Input: dimensioned drawing with shaded views. Units: mm. Origin: part minimum x, y, z. A direction names the side the tool comes from. Round coordinates to 2 decimals unless told otherwise and drop trailing zeros. Loops run counter-clockwise (first coordinate to the right, second up) from the corner with the lowest first, then second, coordinate; pieces in that order, holes last. Notation, with made-up numbers: M 9,33.5 L 38,33.5 A28 cw 38,65.5 Z; hole C -37.5,88.5 d7. An arc over 180 degrees is marked long. Write each question's results on one line, items separated by ' | '. Start each with the question number.
1. Section D-D on x = 5. Output: boundary loops of the cut face in (y, z) (1 decimal).
2. Set-up query: the marked faces 1 and 2. Return all of +Z, -Z, +X, -X, +Y, -Y with unobstructed straight access to the full face (end or side cutting, diameter ignored); none if empty.
3. Contact query for a flat-ended pin moving along its axis: pin 1 Ø4.5 at (y, z) = (25.4, 38.1) entering from +X (1 decimal). Output: stop coordinate, or through.
4. Ray query, line 1 (Y direction, x = 24.5, z = 12.7); line 2 (Y direction, x = 5.5, z = 31) (1 decimal); line 3 (X direction, y = 37, z = 49) (1 decimal). Return the intervals inside material, ascending.
5. Draft query along X for the marked faces 3, 4, 5 and 6. Return one class per face: released by +X, released by -X, zero draft, split by the parting line, or undercut.
6. Section C-C on z = 38.1. Output: boundary loops of the cut face in (x, y) (1 decimal), and give its area (3 significant figures).
7. Section A-A on z = 12.7. Output: boundary loops of the cut face in (x, y) (1 decimal), and give its area (3 significant figures).
8. Section B-B on y = 25.4. Output: boundary loops of the cut face in (x, z) (1 decimal).
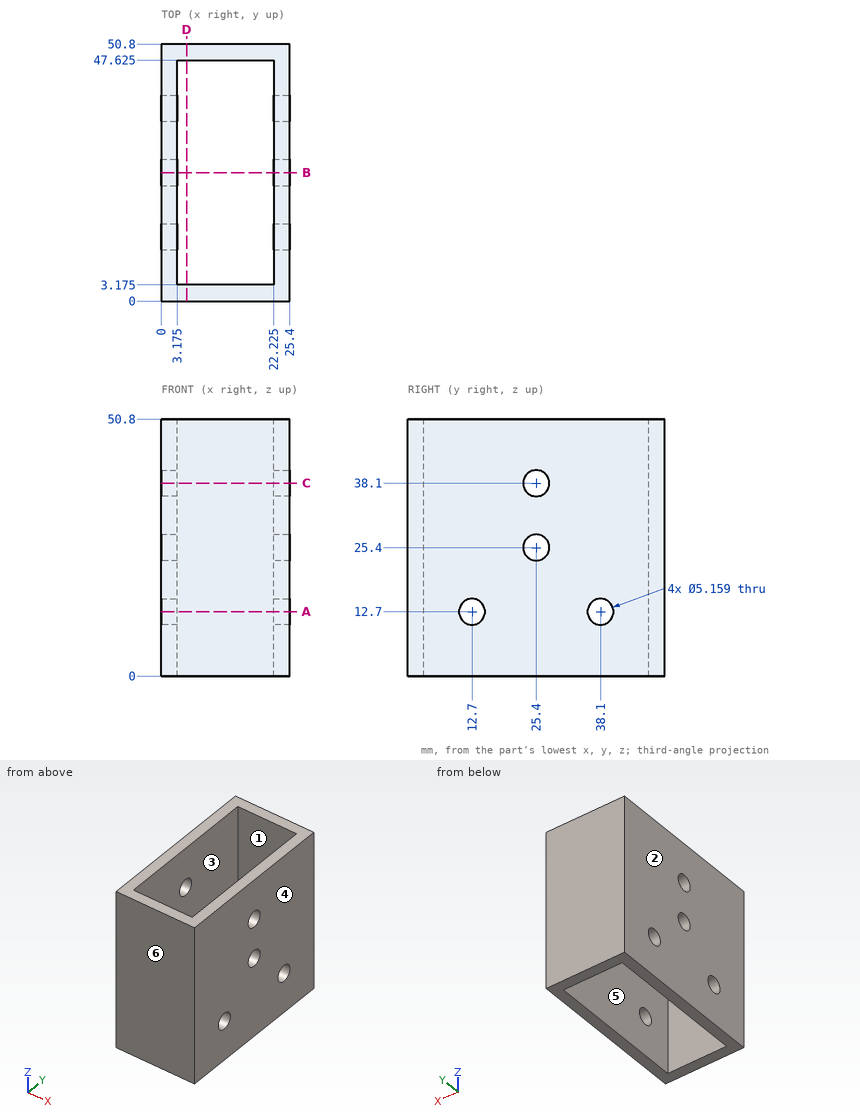
Taken from the geometry:
1) outline: M 0,0 L 3.2,0 L 3.2,50.8 L 0,50.8 Z; M 47.6,0 L 50.8,0 L 50.8,50.8 L 47.6,50.8 Z
2) face 1: +Z, -Z | face 2: +Z, -Z, -X, +Y, -Y
3) pin 1: through
4) line 1: 0 to 10.12, 15.28 to 35.52, 40.68 to 50.8 | line 2: 0 to 3.2, 47.6 to 50.8 | line 3: 0 to 3.2, 22.2 to 25.4
5) face 3: undercut | face 4: released by +X | face 5: undercut | face 6: zero draft
6) outline: M 0,0 L 25.4,0 L 25.4,22.8 L 22.2,22.8 L 22.2,3.2 L 3.2,3.2 L 3.2,22.8 L 0,22.8 Z; M 0,28 L 3.2,28 L 3.2,47.6 L 22.2,47.6 L 22.2,28 L 25.4,28 L 25.4,50.8 L 0,50.8 Z | area: 411 mm^2
7) outline: M 0,0 L 25.4,0 L 25.4,10.1 L 22.2,10.1 L 22.2,3.2 L 3.2,3.2 L 3.2,10.1 L 0,10.1 Z; M 0,15.3 L 3.2,15.3 L 3.2,35.5 L 0,35.5 Z; M 0,40.7 L 3.2,40.7 L 3.2,47.6 L 22.2,47.6 L 22.2,40.7 L 25.4,40.7 L 25.4,50.8 L 0,50.8 Z; M 22.2,15.3 L 25.4,15.3 L 25.4,35.5 L 22.2,35.5 Z | area: 378 mm^2
8) outline: M 0,0 L 3.2,0 L 3.2,22.8 L 0,22.8 Z; M 0,28 L 3.2,28 L 3.2,35.5 L 0,35.5 Z; M 0,40.7 L 3.2,40.7 L 3.2,50.8 L 0,50.8 Z; M 22.2,0 L 25.4,0 L 25.4,22.8 L 22.2,22.8 Z; M 22.2,28 L 25.4,28 L 25.4,35.5 L 22.2,35.5 Z; M 22.2,40.7 L 25.4,40.7 L 25.4,50.8 L 22.2,50.8 Z
